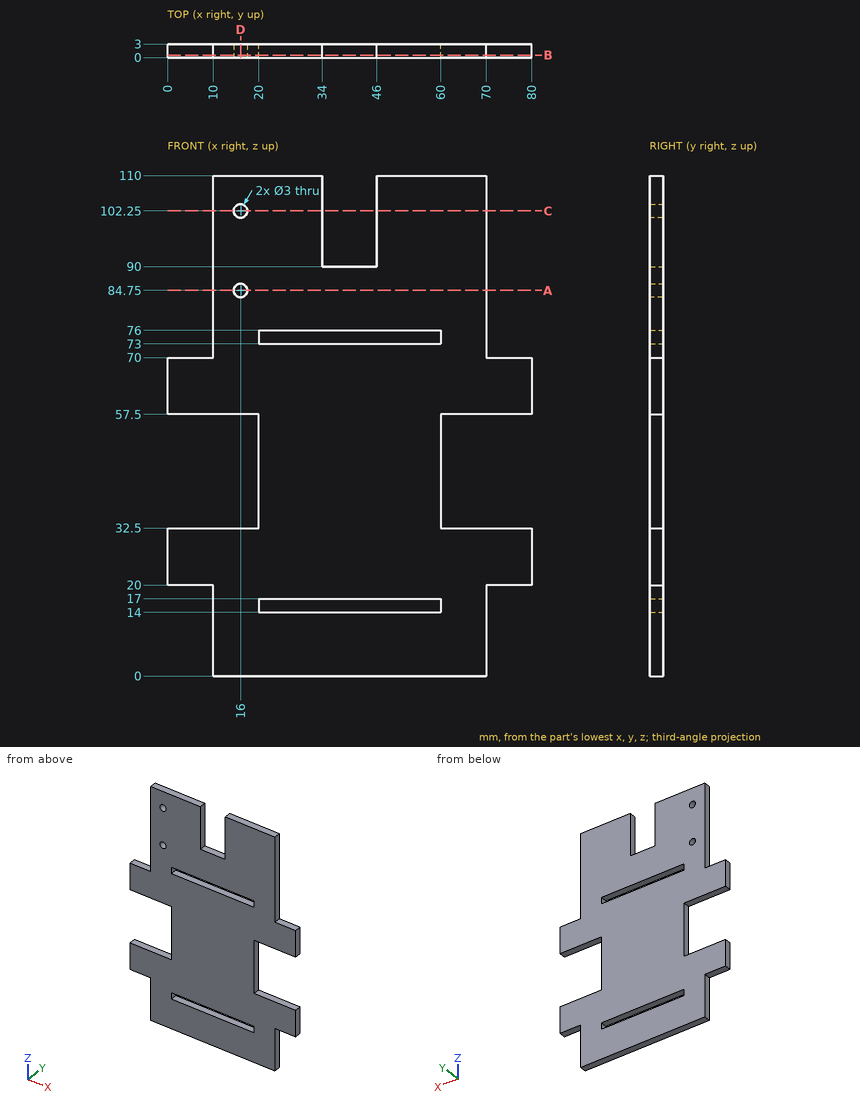
Answer from the drawing. Dimensions are ordinates in mm from the lowest x, y and z of the part. Round coordinates to 2 decimals unless told otherwise and drop trailing zeros. Order: outer loops, then holes, each group sorted by start corner. A loop starts at its lowest first (then second) coordinate and runs counter-clockwise, first axis right, second up. Notation, with made-up numbers: (66.25, -4.5) -> (95.25, -4.5) arc R10 ccw to (95.25, 2.5) -> close; hole circle Ø3 at (-24.75, 39). An arc over 180 degrees is marked (long way). Answer as CSV lines item,"result".
Q1. A cutting plane is placed at B-B on y = 0.55. Give the number of separate pieces and of enclosed holes in the cut face, plus the area to 3 significant figures.
Computed values:
separate pieces,"1"
enclosed holes,"4"
area,"6,110 mm^2"
Q2. A cutting plane is placed at D-D on x = 16. Determine the outline of the cut face in (y, z).
Computed values:
outline,"(0, 0) -> (3, 0) -> (3, 32.5) -> (0, 32.5) -> close; (0, 57.5) -> (3, 57.5) -> (3, 83.25) -> (0, 83.25) -> close; (0, 86.25) -> (3, 86.25) -> (3, 100.75) -> (0, 100.75) -> close; (0, 103.75) -> (3, 103.75) -> (3, 110) -> (0, 110) -> close"
Q3. Consider line 1 (Z direction, x = 27.5, y = 2.7); line 2 (X direction, y = 1.4, z = 102.25); line 3 (Z direction, x = 16, y = 0.6). Determine where each line is inside the solid, lowest interval first. Write a range as from..to.
Computed values:
line 1,"z = 0..14, 17..73, 76..110"
line 2,"x = 10..14.5, 17.5..34, 46..70"
line 3,"z = 0..32.5, 57.5..83.25, 86.25..100.75, 103.75..110"
Q4. A cutting plane is placed at C-C on z = 102.25. Determine the outline of the cut face in (x, y), plus the area to 3 significant figures.
Computed values:
outline,"(10, 0) -> (14.5, 0) -> (14.5, 3) -> (10, 3) -> close; (17.5, 0) -> (34, 0) -> (34, 3) -> (17.5, 3) -> close; (46, 0) -> (70, 0) -> (70, 3) -> (46, 3) -> close"
area,"135 mm^2"
Q5. A cutting plane is placed at A-A on z = 84.75. Determine the outline of the cut face in (x, y), plus the area to 3 significant figures.
Computed values:
outline,"(10, 0) -> (14.5, 0) -> (14.5, 3) -> (10, 3) -> close; (17.5, 0) -> (70, 0) -> (70, 3) -> (17.5, 3) -> close"
area,"171 mm^2"
Q6. Given pin 1 (1.5 mm diameter, centred on y = 1, z = 44.5, fed in from -X); pin 2 (1.5 mm diameter, centred on x = 74.5, y = 2, fed in from +Z); pin 3 (0.9 mm diameter, centred on y = 2, z = 74, fed in from -X), each flat-ended and moving along its own axis, determine where each tip first touches the part or whether it passes through.
Computed values:
pin 1,"stops at x = 20"
pin 2,"stops at z = 70"
pin 3,"stops at x = 10"
